Source: CAD feature listing. Evaluate the final solid. Frame: model axes, mm. A direction names the side the tool comes from. Coordinates: 2 decimals unless noted, no trailing zeros. Loops run counter-clockwise (first coordinate to the right, second up) from the corner with the lowest first, then second, coordinate; pieces in that order, holes last. Notation, with made-up numbers: M 14,23 L 20,23 A37 ccw 20,59 Z; hole C 37,-9.75 d3. An arc over 180 degrees is marked long. One line per question, with ' | ' between items. Start each with the question number.
1. Mould query, pull axis Y, two halves, no side actions, for faces 6 (the cylindrical face through (-0.16, -13.98, 2.96)), 7 (the flat face through (1, -26, 3)), 8 (the cylindrical face through (-10.895, -8.018, 2.958)). Classes: pulls with the +Y half, pulls with the -Y half, needs draft (parallel to the pull), parting line crosses it, or undercut.
2. Pin query (flat end, axial travel): P1, Ø3, axis at y = -26.5, z = 3.5, coming from the +X side; P2, Ø3.5, axis at x = 7.525, y = -11, coming from the -Z side. Return the tip coordinate at first contact, or that it passes through.
3. Section query C-C, the plane y = -11. Output: boundary loops of the cut face in (x, z) (3 decimals).
4. Section query A-A, the plane y = -26.25. Output: boundary loops of the cut face in (x, z), and give its area (3 significant figures).
5. Access query for faces 1 (the flat face through (-4, -27, 3)), 2 (the flat face through (0, -13, 0)), 3 (the cylindrical face through (2.254, -9.853, 2.958)), 4 (the flat face through (4, -27, 3)), 5 (the flat face through (-1, -26, 3)). Directions: +Z, -Z, +X, -X, +Y, -Y. A direction counts if a zero-diameter tool reaches every point of the face in a straight line with its end or side. Return the directions, or none.
6. Section query D-D, the plane y = -18. Output: boundary loops of the cut face in (x, z) (3 decimals).
7. Ray query, probe 1 along X at (y, z) = (-27.5, 2.55); probe 2 along X at (y, z) = (-9.5, 0.75); probe 3 along X at (y, z) = (-11.5, 5.1). Return the intervals inside material, ascending.
8. Section query B-B, the plane z = 1.8. State how many separate pieces and enclosed holes the cut face has, and give its area (3 significant figures).
Autodesk Inventor part; units mm, degrees
ref_plane "YZ Plane" through (0, 0, 0) normal (1, 0, 0) x (0, 1, 0)
ref_plane "XZ Plane" through (0, 0, 0) normal (0, 1, 0) x (-1, 0, 0)
ref_plane "XY Plane" through (0, 0, 0) normal (0, 0, 1) x (1, 0, 0)
sketch "スケッチ1" plane through (0, 0, 0) normal (0, 0, 1) x (1, 0, 0)
  circle A0 centre (0, 0) radius 4.025
  arc A1 (6.725498, 2.029361) -> (-6.725498, 2.029361) centre (0, 0) ccw
  line L0 (0, -11) -> (0, -19) construction
  line L1 (-3.025, -11) -> (-3.025, -19)
  line L2 (3.025, -19) -> (3.025, -11)
  arc A2 (3.025, -11) -> (-3.025, -11) centre (0, -11) ccw
  arc A3 (-3.025, -19) -> (3.025, -19) centre (0, -19) ccw
  arc A4 (-5.235739, -21.981218) -> (5.235739, -21.981218) centre (0, -19) ccw
  circle A5 centre (-7.525, -11) radius 1.25
  circle A6 centre (7.525, -11) radius 1.25
  line L3 (-7.525, -11) -> (7.525, -11) construction
  arc A7 (-11.411415, -8.73157) -> (-10.923603, -13.949491) centre (-7.525, -11) ccw
  arc A8 (-11.411415, -8.73157) -> (-6.725498, 2.029361) centre (-54.593809, 16.473208) ccw
  arc A9 (6.725498, 2.029361) -> (11.411415, -8.73157) centre (54.593809, 16.473208) ccw
  arc A10 (-5.235739, -21.981218) -> (-10.923603, -13.949491) centre (-48.685856, -46.721617) ccw
  arc A11 (10.923603, -13.949491) -> (5.235739, -21.981218) centre (48.685856, -46.721617) ccw
  arc A12 (10.923603, -13.949491) -> (11.411415, -8.73157) centre (7.525, -11) ccw
  point P0 (0, -15)
  dimension "d0" = 8.05
  dimension "d1" = 3
  dimension "d2" = 8
  dimension "d3" = 6.05
  dimension "d4" = 19
  dimension "d5" = 2.5
  dimension "d6" = 2.5
  dimension "d7" = 9
  dimension "d8" = 100
  dimension "d9" = 100
  dimension "d10" = 50
  dimension "d11" = 50
  dimension "d12" = 4.5
  dimension "d13" = 3
sketch "スケッチ2" plane through (0, 0, 0) normal (0, 0, 1) x (1, 0, 0)
  circle A0 centre (-7.525, -11) radius 1.25 construction
  circle A1 centre (7.525, -11) radius 1.25 construction
  circle A2 centre (-7.525, -11) radius 2
  circle A3 centre (7.525, -11) radius 2
  arc A4 (-3.027118, -11.138035) -> (-7.062601, -15.47618) centre (-7.525, -11) ccw
  arc A5 (7.062601, -15.47618) -> (3.027118, -11.138035) centre (7.525, -11) ccw
  arc A6 (1, -21.898798) -> (-1, -21.898798) centre (0, -18) ccw
  line L0 (0, 0) -> (0, -18) construction
  line L1 (-1, -21.898798) -> (-1, -29.898798)
  line L2 (1, -21.898798) -> (1, -29.898798)
  line L3 (1, -29.898798) -> (4, -29.898798)
  line L4 (4, -29.898798) -> (4, -24.344289)
  line L5 (-1, -29.898798) -> (-4, -29.898798)
  line L6 (-4, -29.898798) -> (-4, -24.344289)
  arc A7 (-7.062601, -15.47618) -> (-4, -24.344289) centre (0, -18) ccw
  arc A8 (4, -24.344289) -> (7.062601, -15.47618) centre (0, -18) ccw
  arc A9 (3.027118, -11.138035) -> (-3.027118, -11.138035) centre (0, -18) ccw
  dimension "d14" = 4
  dimension "d15" = 4
  dimension "d16" = 9
  dimension "d17" = 9
  dimension "d18" = 8.05
  dimension "d19" = 18
  dimension "d20" = 8
  dimension "d21" = 8
  dimension "d22" = 2
  dimension "d23" = 1
  dimension "d24" = 3
  dimension "d25" = 3
  dimension "d27" = 7.5
  dimension "d28" = 7.5
  dimension "d29" = 7.5
sketch "スケッチ2 outline for 押し出し1" plane through (0, 0, 0) normal (0, 0, 1) x (1, 0, 0)
  line L0 (-1, -29.898798) -> (-1, -21.898798)
  line L1 (-4, -29.898798) -> (-1, -29.898798)
  arc A0 (-1, -21.898798) -> (1, -21.898798) centre (0, -18) cw
  line L2 (-4, -24.344289) -> (-4, -29.898798)
  line L3 (1, -21.898798) -> (1, -29.898798)
  arc A1 (-7.062601, -15.47618) -> (-4, -24.344289) centre (0, -18) ccw
  line L4 (1, -29.898798) -> (4, -29.898798)
  arc A2 (-3.027118, -11.138035) -> (-7.062601, -15.47618) centre (-7.525, -11) ccw
  line L5 (4, -29.898798) -> (4, -24.344289)
  arc A3 (3.027118, -11.138035) -> (-3.027118, -11.138035) centre (0, -18) ccw
  arc A4 (4, -24.344289) -> (7.062601, -15.47618) centre (0, -18) ccw
  arc A5 (7.062601, -15.47618) -> (3.027118, -11.138035) centre (7.525, -11) ccw
  circle A6 centre (-7.525, -11) radius 2
  circle A7 centre (7.525, -11) radius 2
extrude "押し出し1" add sketch "スケッチ2 outline for 押し出し1" along normal blind 6
fillet "フィレット1" radius 5 4 edges at (-3.0271, -11.138, 3) (3.0271, -11.138, 3) (7.0626, -15.4762, 3) (-7.0626, -15.4762, 3)
equation "\"d21\" = d20"
properties part number "横回転棒取り付けパーツ" material "アルミニウム 7075"
Taken from the geometry:
1) face 6: undercut | face 7: needs draft | face 8: parting line crosses it
2) P1: x = 4 | P2: through
3) outline: M -12.025,0 L -9.525,0 L -9.525,6 L -12.025,6 Z; M -5.525,0 L 5.525,0 L 5.525,6 L -5.525,6 Z; M 9.525,0 L 12.025,0 L 12.025,6 L 9.525,6 Z
4) outline: M -4,0 L -1,0 L -1,6 L -4,6 Z; M 1,0 L 4,0 L 4,6 L 1,6 Z | area: 36.0 mm^2
5) face 1: +Z, -Z, -X, -Y | face 2: -Z, +X, -X, +Y, -Y | face 3: +Z, -Z, +Y | face 4: +Z, -Z, +X, -Y | face 5: +Z, -Z, -Y
6) outline: M -7.577,0 L -4.025,0 L -4.025,6 L -7.577,6 Z; M 4.025,0 L 7.577,0 L 7.577,6 L 4.025,6 Z
7) probe 1: -4 to -1, 1 to 4 | probe 2: -11.77 to -8.85, -6.2 to -2.78, 2.79 to 6.2, 8.85 to 11.77 | probe 3: -12 to -9.46, -5.59 to 5.59, 9.46 to 12
8) separate pieces: 1 | enclosed holes: 2 | area: 245 mm^2
